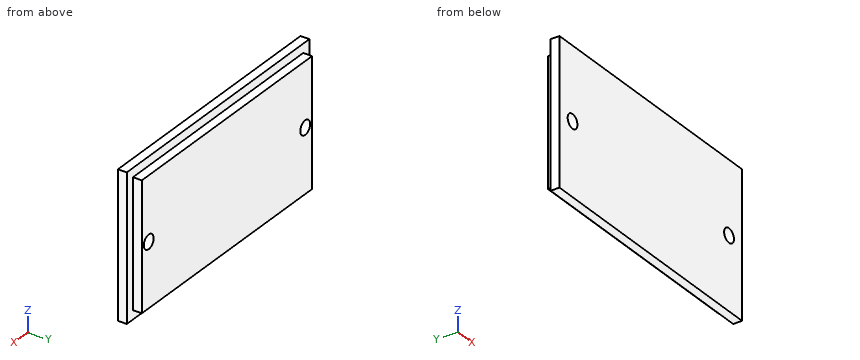
from build123d import *

# Parameters (mm, degrees)
F0_W     = 49.6
F0_H     = 25.7
F0_R     = 1.425
F1_DEPTH = 3.6
F0_W_2   = 53.2
F0_H_2   = 29.3
F2_DEPTH = 1.8


with BuildPart() as f1:
    # F0 (on Front) → F1 (new body)
    with BuildSketch(Plane.XZ):
        Rectangle(F0_W, F0_H)
        with Locations((-22.8, 0)):
            Circle(F0_R, mode=Mode.SUBTRACT)
        with Locations((22.8, 0)):
            Circle(F0_R, mode=Mode.SUBTRACT)
    extrude(amount=-F1_DEPTH)

    # F0 (on Front) → F2 (join)
    with BuildSketch(Plane.XZ):
        Rectangle(F0_W_2, F0_H_2)
        Rectangle(F0_W, F0_H, mode=Mode.SUBTRACT)
    extrude(amount=-F2_DEPTH)


solid = f1.part
For this review, take the finished solid that the model builds, in its own axes (mm). Round coordinates to 2 decimals unless told otherwise and drop trailing zeros. Loops run counter-clockwise (first coordinate to the right, second up) from the corner with the lowest first, then second, coordinate; pieces in that order, holes last. Notation, with made-up numbers: (11.5, 68) - (59.5, 68) arc R21 ccw to (59.5, 97) - close; hole circle Ø2 at (-19.75, 74.5). An arc over 180 degrees is marked (long way). One line per question, with ' | ' between items.
Q1. Take a section at D-D (x = -7.5). Give the boundary of the cut face in (y, z), and give its area (3 significant figures).
Taken from the geometry:
outline: (0, -14.65) - (1.8, -14.65) - (1.8, -12.85) - (3.6, -12.85) - (3.6, 12.85) - (1.8, 12.85) - (1.8, 14.65) - (0, 14.65) - close | area: 99.0 mm²
Q2. For line 1 along Z through (x, y) = (-22.8, 1.15) (3 decimals); line 2 along Z through (x, y) = (22.8, 2.85) (3 decimals); line 3 along X through (y, z) = (2.15, 0.5), list the stretches that pass through material, from the lowest coordinate up. Write a range as [from, to].
Taken from the geometry:
line 1: z = [-14.65, -1.425], [1.425, 14.65] | line 2: z = [-12.85, -1.425], [1.425, 12.85] | line 3: x = [-24.8, -24.13], [-21.47, 21.47], [24.13, 24.8]
Q3. Take a section at C-C (z = -11). Give the boundary of the cut face in (x, y), and give its area (3 significant figures).
Taken from the geometry:
outline: (-26.6, 0) - (26.6, 0) - (26.6, 1.8) - (24.8, 1.8) - (24.8, 3.6) - (-24.8, 3.6) - (-24.8, 1.8) - (-26.6, 1.8) - close | area: 185 mm²
Q4. Take a section at B-B (x = 22.8). Give the boundary of the cut face in (y, z) (3 decimals).
Taken from the geometry:
outline: (0, -14.65) - (1.8, -14.65) - (1.8, -12.85) - (3.6, -12.85) - (3.6, -1.425) - (0, -1.425) - close; (0, 1.425) - (3.6, 1.425) - (3.6, 12.85) - (1.8, 12.85) - (1.8, 14.65) - (0, 14.65) - close
Q5. Take a section at A-A (z = 0). Give the boundary of the cut face in (x, y) (3 decimals), and give its area (3 significant figures).
Taken from the geometry:
outline: (-26.6, 0) - (-24.225, 0) - (-24.225, 3.6) - (-24.8, 3.6) - (-24.8, 1.8) - (-26.6, 1.8) - close; (-21.375, 0) - (21.375, 0) - (21.375, 3.6) - (-21.375, 3.6) - close; (24.225, 0) - (26.6, 0) - (26.6, 1.8) - (24.8, 1.8) - (24.8, 3.6) - (24.225, 3.6) - close | area: 165 mm²
Q6. For pin 1 (10 mm diameter, centred on x = 10.5, z = -4.5, fed in from -Y); pin 2 (2.5 mm diameter, centred on x = 22.8, z = 0, fed in from -Y); pin 3 (0.5 mm diameter, centred on x = -8.5, y = 2.5, fed in from +Z), all flat-tipped, find the tip position at first contact; note any pin that passes through.
Taken from the geometry:
pin 1: stops at y = 0 | pin 2: passes through | pin 3: stops at z = 12.85
